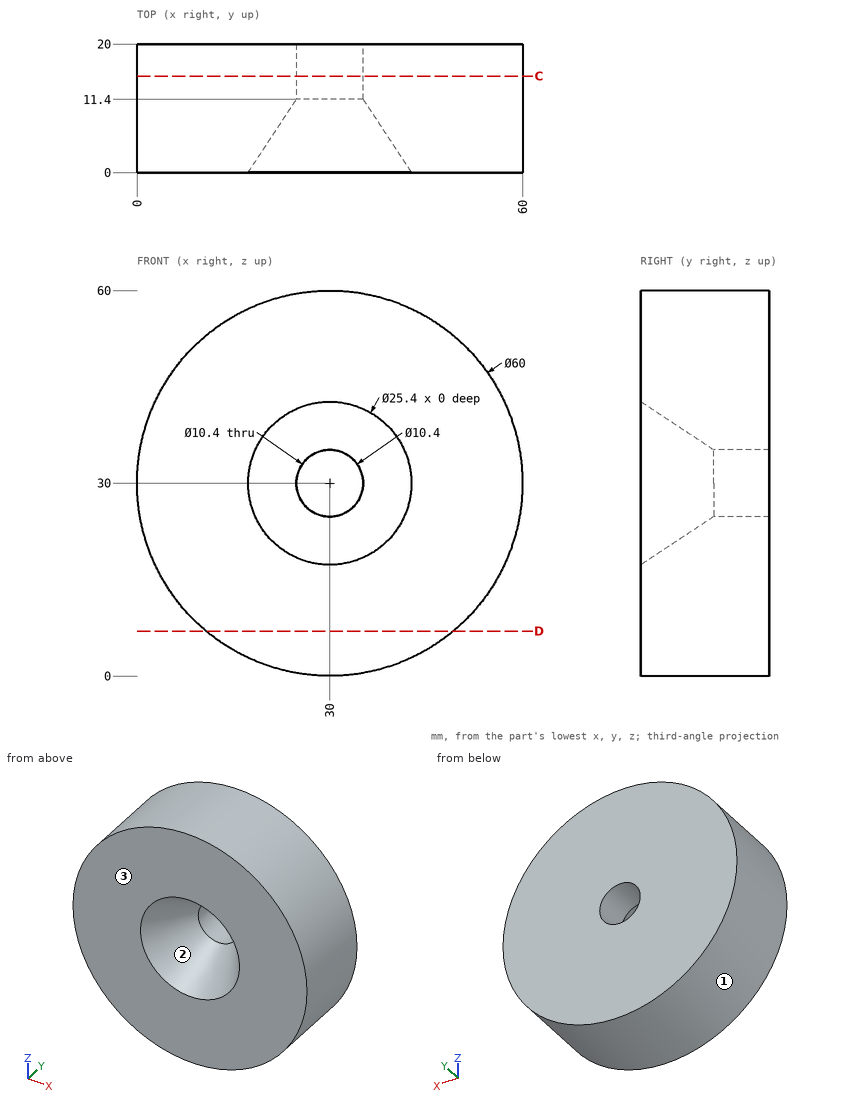
For this review, use the dimensioned drawing (mm, ordinates from the lowest corner) and the shaded views. Give positions to 0.01 mm unless a question says otherwise; leave off trailing zeros. Write each loop counter-clockwise with the first axis right and the second up, starting at its lowest first coordinate (ties: lowest second). Pieces come first, ordered by that corner, then holes.
(1) Consider section D-D, the plane z = 7. Give the boundary of the cut face in (x, y).
(2) Consider section C-C, the plane y = 15. Give the boundary of the cut face in (x, z), and give its area (3 significant figures).
(3) For P1, Ø10, axis at x = 46.5, y = 13.5, coming from the +Z side; P2, Ø6, axis at x = 30.5, y = 4.5, coming from the -Z side; P3, Ø8, axis at x = 22, y = 18, coming from the +Z side, all flat-tipped, find the tip position at first contact; note any pin that passes through.
(4) The part is to be moulded in two halves that separate along Z. For the marked faces 1, 2 and 3, say which applies: released by +Z, released by -Z, zero draft, split by the parting line, or undercut.
(5) To check wall thickness, follow L1, parallel to Z at x = 30, y = 14.25; L2, parallel to X at y = 8.5, z = 26 (1 decimal); L3, parallel to Z at x = 30, y = 0.05. State the ranges of each line that lie inside material, in increasing order.
Returned:
1. outline: (10.74, 0) - (49.26, 0) - (49.26, 20) - (10.74, 20) - close
2. outline: circle Ø60 at (30, 30); hole circle Ø10.4 at (30, 30)
2. area: 2,740 mm2
3. P1: stops at z = 57.71
3. P2: stops at z = 0
3. P3: stops at z = 59.73
4. face 1: split by the parting line
4. face 2: undercut
4. face 3: zero draft
5. L1: z = 0 to 24.8, 35.2 to 60
5. L2: x = 0.3 to 24.1, 35.9 to 59.7
5. L3: z = 0 to 17.33, 42.67 to 60
